Work out the finished part from the listing and answer in its coordinate system (mm). A direction names the side the tool comes from. Round coordinates to 2 decimals unless told otherwise and drop trailing zeros. Order: outer loops, then holes, each group sorted by start corner. A loop starts at its lowest first (then second) coordinate and runs counter-clockwise, first axis right, second up.
from build123d import *

# Parameters (mm, degrees)
BOSS_EXTRUDE1_DEPTH      = 18.75
SKETCH4_W                = 36.15
SKETCH4_H                = 12.5
CUT_EXTRUDE1_DEPTH       = 5
CUT_EXTRUDE2_DEPTH       = 6
CUT_EXTRUDE2_DEPTH_BACK  = 4.5
SKETCH6_R                = 1.5
CUT_EXTRUDE3_DEPTH       = 60.223179584
SKETCH7_W                = 2
SKETCH7_H                = 4.5
SKETCH7_W_2              = 1.25
CUT_EXTRUDE4_DEPTH       = 3
SKETCH7_3_W              = 1.25
SKETCH7_3_H              = 2.5
CUT_EXTRUDE5_DEPTH       = 5
CUT_EXTRUDE6_DEPTH       = 9.5
SKETCH9_W                = 7.25
SKETCH9_H                = 6.25
BOSS_EXTRUDE2_DEPTH      = 5.75
CUT_EXTRUDE7_DEPTH       = 9.5
CUT_EXTRUDE8_DEPTH       = 12
CUT_EXTRUDE8_DEPTH_BACK  = 54.706470746
CUT_EXTRUDE11_DEPTH      = 6
CUT_EXTRUDE11_DEPTH_BACK = 2.75
SKETCH12_W               = 15.15
SKETCH12_H               = 4.7
SKETCH13_R               = 1.25
CUT_EXTRUDE12_DEPTH      = 58.496825999


with BuildPart() as part:
    # Sketch1 → Boss-Extrude1 (new body)
    with BuildSketch(Plane.XY):
        with BuildLine():
            Line((11.5, 3.5), (11.5, 11))
            Line((11.5, 11), (30.75, 11))
            Line((30.75, 11), (30.75, -1))
            ThreePointArc((30.75, -1), (26.002013283, -12.110227589), (28.15, -24))
            Line((28.15, -24), (36.15, -31))
            Line((36.15, -31), (36.15, -43))
            Line((36.15, -43), (10, -43))
            Line((10, -43), (10, -34.5))
            Line((10, -34.5), (5, -30.5))
            Line((5, -30.5), (0, -30.5))
            Line((0, -30.5), (0, 0))
            Line((0, 0), (6.5, 3.5))
            Line((6.5, 3.5), (11.5, 3.5))
        make_face()
    extrude(amount=BOSS_EXTRUDE1_DEPTH)

    # Sketch4 → Cut-Extrude1 (cut)
    with BuildSketch(Plane(origin=(0, 0, 0), x_dir=(-1, 0, 0), z_dir=(0, 0, -1))):
        with Locations((-18.075, -36.75)):
            Rectangle(SKETCH4_W, SKETCH4_H)
    extrude(amount=-CUT_EXTRUDE1_DEPTH, mode=Mode.SUBTRACT)

    # Sketch5 → Cut-Extrude2 (cut, two sides: drawn at the far end of the back side and taken through both)
    with BuildSketch(Plane(origin=(0, 0, 5), x_dir=(-1, 0, 0), z_dir=(0, 0, -1)).offset(-CUT_EXTRUDE2_DEPTH_BACK)):
        Polygon((-32.35, -43), (-13.8, -43), (-13.8, -37), (0.902131261, -37), (0.902131261, -29.5), (-36.15, -29.5), (-36.15, -37), (-32.35, -37), align=None)
    extrude(amount=CUT_EXTRUDE2_DEPTH + CUT_EXTRUDE2_DEPTH_BACK, mode=Mode.SUBTRACT)

    # Sketch6 → Cut-Extrude3 (cut, through all)
    with BuildSketch(Plane(origin=(36.15, 0, 0), x_dir=(0, 0, -1), z_dir=(1, 0, 0))):
        with Locations(Location((-8, -40, 0), (0, 0, 90))):
            Circle(SKETCH6_R)
    extrude(amount=-CUT_EXTRUDE3_DEPTH, mode=Mode.SUBTRACT)

    # Sketch7 → Cut-Extrude4 (cut)
    with BuildSketch(Plane(origin=(0, 0, 0), x_dir=(-1, 0, 0), z_dir=(0, 0, -1))):
        with Locations((-27.575, -27.25)):
            Rectangle(SKETCH7_W, SKETCH7_H)
        with Locations((-8.95, -27.25)):
            Rectangle(SKETCH7_W_2, SKETCH7_H)
    extrude(amount=-CUT_EXTRUDE4_DEPTH, mode=Mode.SUBTRACT)

    # Sketch7<3> → Cut-Extrude5 (cut)
    with BuildSketch(Plane(origin=(0, 0, 0), x_dir=(-1, 0, 0), z_dir=(0, 0, -1))):
        with Locations((-8.95, -8.75)):
            Rectangle(SKETCH7_3_W, SKETCH7_3_H)
        with BuildLine():
            ThreePointArc((-27.058287436, -7.5), (-26.801337311, -8.279605972), (-26.575, -9.068643524))
            Line((-26.575, -9.068643524), (-26.575, -7.5))
            Line((-26.575, -7.5), (-27.058287436, -7.5))
        make_face()
    extrude(amount=-CUT_EXTRUDE5_DEPTH, mode=Mode.SUBTRACT)

    # Sketch8 → Cut-Extrude6 (cut)
    with BuildSketch(Plane(origin=(0, 0, 0), x_dir=(-1, 0, 0), z_dir=(0, 0, -1))):
        Polygon((-8.325, -10), (-8.325, -7.5), (-33.629917385, -7.5), (-33.629917385, 11), (0, 11), (0, -30.5), (-8.325, -30.5), (-8.325, -25), (-9.575, -25), (-9.575, -10), align=None)
    extrude(amount=-CUT_EXTRUDE6_DEPTH, mode=Mode.SUBTRACT)

    # Sketch9 → Boss-Extrude2 (add)
    with BuildSketch(Plane(origin=(0, 0, 9.5), x_dir=(-1, 0, 0), z_dir=(0, 0, -1))):
        with Locations((-15.125, 7.875)):
            Rectangle(SKETCH9_W, SKETCH9_H)
    extrude(amount=BOSS_EXTRUDE2_DEPTH)

    # Sketch10 → Cut-Extrude7 (cut)
    with BuildSketch(Plane(origin=(0, 0, 0), x_dir=(-1, 0, 0), z_dir=(0, 0, -1))):
        Polygon((-35.578571429, -29.5), (-28.575, -29.5), (-28.575, -25), (-26.356090024, -25), (-26.356090024, -9.972017094), (-27.488550882, -9.972017094), (-27.488550882, -22.567234298), (-35.578571429, -22.567234298), align=None)
    extrude(amount=-CUT_EXTRUDE7_DEPTH, mode=Mode.SUBTRACT)

    # Sketch11 → Cut-Extrude8 (cut, two sides: drawn at the far end of the back side and taken through both)
    with BuildSketch(Plane.ZY.offset(-10).offset(-CUT_EXTRUDE8_DEPTH_BACK)):
        Polygon((12.25, -43), (18.75, -43), (18.75, -29), (12.25, -33.7), align=None)
    extrude(amount=CUT_EXTRUDE8_DEPTH + CUT_EXTRUDE8_DEPTH_BACK, mode=Mode.SUBTRACT)

    # Sketch12 → Cut-Extrude11 (cut, two sides: drawn at the far end of the back side and taken through both)
    with BuildSketch(Plane.XY.offset(12.25).offset(-CUT_EXTRUDE11_DEPTH_BACK)):
        with Locations((19.575, -31.35)):
            Rectangle(SKETCH12_W, SKETCH12_H)
    extrude(amount=CUT_EXTRUDE11_DEPTH + CUT_EXTRUDE11_DEPTH_BACK, mode=Mode.SUBTRACT)

    # Sketch13 → Cut-Extrude12 (cut, through all)
    with BuildSketch(Plane.XY.offset(12.25)):
        with Locations((23.075, -36.2)):
            Circle(SKETCH13_R)
    extrude(amount=-CUT_EXTRUDE12_DEPTH, mode=Mode.SUBTRACT)


solid = part.part
Item 1: Find section D-D (z = 14.5). Write down the section's boundary in (x, y), plus the area to 3 significant figures.
Item 2: Find the intervals of material crossed by line 1 along Z through (x, y) = (12.55, -40); line 2 along Z through (x, y) = (7.5, -13); line 3 along Y through (x, z) = (15.5, 11), in increasing order.
Item 3: A tool of negligible diameter and unlimited length cuts with its end or side. For faces 5 (the face through (15, 8, 3.75)), 6 (the face through (9, -10, 7)), 7 (the face through (9, -27, 3)), 8 (the face through (27, -25, 6)), from which of +Z, -Z, +X, -X, +Y, -Y can it reach the whole face along a straight path? Write none if from no direction.
Item 4: For a pull along Y with two mould halves and no side action, classify faces 1 (the face through (26.356, -22, 5)), 2 (the face through (27.15, -31, 13)), 3 (the face through (34, -37, 7)), 4 (the face through (17, -9, 18.75)) as released by +Y, released by -Y, zero draft, split by the parting line, or undercut.
Item 5: Find section A-A (x = 17.5). Write down the section's boundary in (y, z), plus the area to 3 significant figures.
Item 6: Given pin 1 (1.5 mm diameter, centred on x = 27.5, z = 7, fed in from -Y); pin 2 (1.7 mm diameter, centred on y = -8, z = 1.5, fed in from +X) (3 decimals); pin 3 (1 mm diameter, centred on y = -20.5, z = 6.5, fed in from +X), each flat-ended and moving along its own axis, determine where each tip first touches the part or whether it passes through.
Item 7: Find section B-B (y = -36.2). Write down the section's boundary in (x, z) (3 decimals).
Item 8: Find section C-C (z = 8). State how many separate pieces and enclosed holes the cut face has, plus the area to 3 significant figures.
Model answer:
1. outline: (0, -30.5) - (5, -30.5) - (6.97, -32.07) - (12, -32.07) - (12, -29) - (27.15, -29) - (27.15, -32.07) - (36.15, -32.07) - (36.15, -31) - (28.15, -24) arc R21.03 cw to (30.75, -1) - (30.75, 11) - (11.5, 11) - (11.5, 3.5) - (6.5, 3.5) - (0, 0) - close
1. area: 1,100 mm2
2. line 1: z = 5 to 6.5, 9.5 to 12.25
2. line 2: z = 9.5 to 18.75
2. line 3: y = -43 to -33.7, -29 to 11
3. face 5: -Z, +X, -X, +Y
3. face 6: -Z, -X
3. face 7: -Z, -X, +Y, -Y
3. face 8: -Z, +X
4. face 1: undercut
4. face 2: undercut
4. face 3: released by +Y
4. face 4: zero draft
5. outline: (-43, 9.5) - (-33.7, 9.5) - (-33.7, 12.25) - (-43, 12.25) - close; (-29.5, 0) - (-7.5, 0) - (-7.5, 9.5) - (4.75, 9.5) - (4.75, 3.75) - (11, 3.75) - (11, 18.75) - (-29, 18.75) - (-29.36, 18.25) - (-29, 18.25) - (-29, 9.5) - (-29.5, 9.5) - close
5. area: 641 mm2
6. pin 1: stops at y = -29.5
6. pin 2: stops at x = 26.575
6. pin 3: stops at x = 26.36
7. outline: (10, 9.5) - (21.825, 9.5) - (21.825, 12.25) - (10, 12.25) - close; (24.325, 9.5) - (36.15, 9.5) - (36.15, 12.25) - (24.325, 12.25) - close
8. separate pieces: 6
8. enclosed holes: 0
8. area: 454 mm2
